Verification items for this drawing (mm, ordinates from the low corner). A direction names the side the tool comes from. Coordinates: 2 decimals unless noted, no trailing zeros. Loops run counter-clockwise (first coordinate to the right, second up) from the corner with the lowest first, then second, coordinate; pieces in that order, holes last.
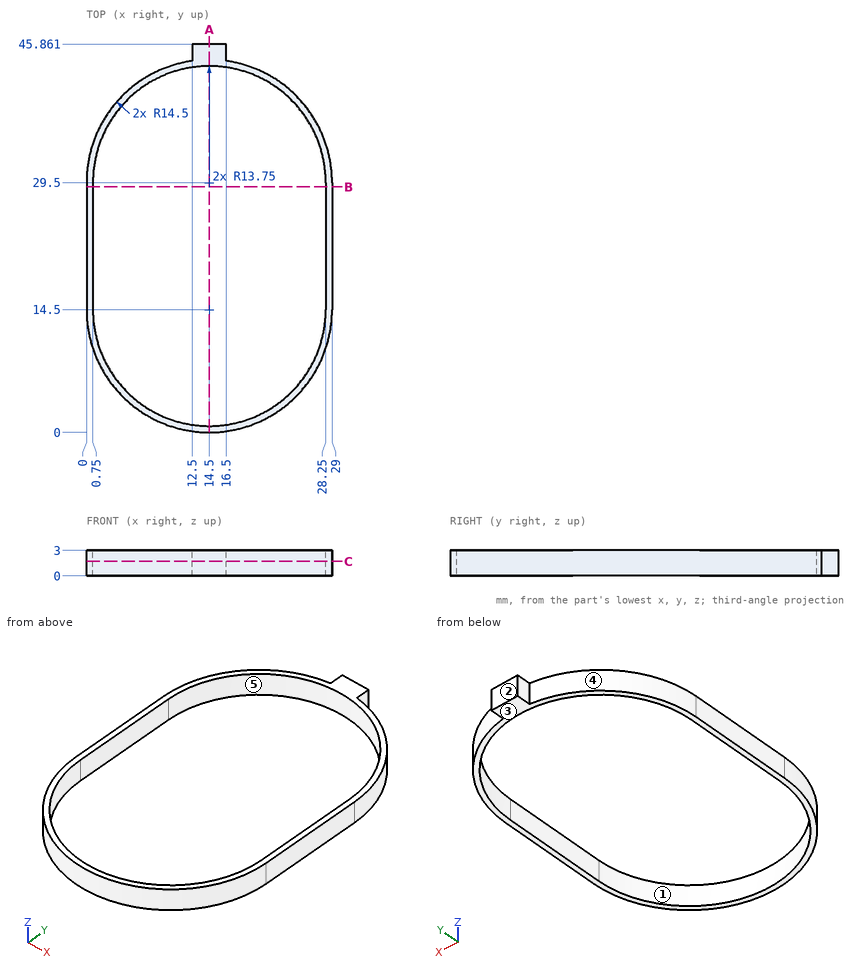
(1) Draft check along X on the marked faces 3, 4 and 5. Enter one of: pulls with the +X half, pulls with the -X half, needs draft (parallel to the pull), parting line crosses it, or undercut.
(2) Section check B-B, the plane y = 29. Enter the section's corners in (x, z).
(3) Set-up check for the marked faces 1 and 2: record each of +Z, -Z, +X, -X, +Y, -Y from which the full face is reachable in a straight line by a thin tool's end or side.
(4) Section check A-A, the plane x = 14.5. Enter the section's corners in (y, z), plus the area to 3 significant figures.
(5) Scan lines: line 1 along X through (y, z) = (15.5, 2.4); line 2 along X through (y, z) = (33, 1); line 3 along Y through (x, z) = (20.75, 0.5) (1 decimal). Record each from-to range of solid material in increasing order.
(6) Gauge pin test, flat ends, axial feed: P1, Ø0.6, axis at y = 45, z = 1.5, coming from the +X side; P2, Ø1.6, axis at y = 45.5, z = 1, coming from the -X side. Record the tip position at first contact, or that the pin passes through.
(7) Section check C-C, the plane z = 1.7. Enter the section's corners in (x, y).
Determined:
1. face 3: needs draft
1. face 4: pulls with the -X half
1. face 5: undercut
2. outline: (0, 0) - (0.75, 0) - (0.75, 3) - (0, 3) - close; (28.25, 0) - (29, 0) - (29, 3) - (28.25, 3) - close
3. face 1: +Z, -Z
3. face 2: +Z, -Z, +X, -X, +Y
4. outline: (0, 0) - (0.75, 0) - (0.75, 3) - (0, 3) - close; (43.25, 0) - (45.86, 0) - (45.86, 3) - (43.25, 3) - close
4. area: 10.1 mm2
5. line 1: x = 0 to 0.75, 28.25 to 29
5. line 2: x = 0.43 to 1.2, 27.8 to 28.57
5. line 3: y = 1.4 to 2.3, 41.7 to 42.6
6. P1: stops at x = 16.5
6. P2: stops at x = 12.5
7. outline: (0, 14.5) arc R14.5 ccw to (29, 14.5) - (29, 29.5) arc R14.5 ccw to (16.5, 43.86) - (16.5, 45.86) - (12.5, 45.86) - (12.5, 43.86) arc R14.5 ccw to (0, 29.5) - close; hole (0.75, 14.5) arc R13.75 ccw to (28.25, 14.5) - (28.25, 29.5) arc R13.75 ccw to (0.75, 29.5) - close
